from build123d import *

# Parameters (mm, degrees)
SKETCH1_R                = 5
BOSS_EXTRUDE1_DEPTH      = 1.5
BOSS_EXTRUDE1_DEPTH_BACK = 1.5


with BuildPart() as part:
    # Sketch1 → Boss-Extrude1 (new body, two sides)
    with BuildSketch(Plane.XY) as boss_extrude1_sk:
        with BuildLine():
            Line((-12.7, 0), (-12.7, -30.012513048))
            Line((-12.7, -30.012513048), (-11.2, -30.012513048))
            ThreePointArc((-11.2, -30.012513048), (0, -23.3), (11.2, -30.012513048))
            Line((11.2, -30.012513048), (12.7, -30.012513048))
            Line((12.7, -30.012513048), (12.7, 0))
            ThreePointArc((12.7, 0), (0, 12.7), (-12.7, 0))
        make_face()
        Circle(SKETCH1_R, mode=Mode.SUBTRACT)
    extrude(amount=BOSS_EXTRUDE1_DEPTH)
    extrude(boss_extrude1_sk.sketch, amount=-BOSS_EXTRUDE1_DEPTH_BACK)


solid = part.part
The listing builds one solid part. Answer for the finished solid, in the listing's coordinates (mm). Round coordinates to 2 decimals unless told otherwise and drop trailing zeros. Write each loop counter-clockwise with the first axis right and the second up, starting at its lowest first coordinate (ties: lowest second). Pieces come first, ordered by that corner, then holes. Notation, with made-up numbers: M -4.5,-6.5 L 37.5,-6.5 A23 ccw 37.5,29.5 Z; hole C -36.5,-31.5 d8. An arc over 180 degrees is marked long. Write each question's results on one line, items separated by ' | '. Start each with the question number.
(1) The part is cut by section A-A, the plane z = -0.05. Write down the section's boundary in (x, y).
(2) This flat-tipped pin is pushed along its axis until it touches: P1, Ø1, axis at y = 3.5, z = 0, coming from the +X side. Where does it stop, or does it pass through?
(3) The part is cut by section B-B, the plane x = 0. Write down the section's boundary in (y, z), and give its area (3 significant figures).
(4) The part is cut by section D-D, the plane y = 7.5. Write down the section's boundary in (x, z).
(5) Find the intervals of material crossed by line 1 (X direction, y = -27.5, z = -1.15); line 2 (Y direction, x = 4, z = -0.55); line 3 (X direction, y = 1, z = -0.45), in increasing order.
(6) Determine the mould class of faces 1 (the cylindrical face through (-1.08, -4.88, -0.02)), 2 (the flat face through (12, -30.013, 0)), 3 (the flat face through (12.7, -15, 0)) for opening direction Y: +Y half, -Y half, draft (parallel to the pull), parting line (faces both ways), or undercut.
(7) The part is cut by section C-C, the plane y = 1.5. Write down the section's boundary in (x, z), and give its area (3 significant figures).
Worked answers:
1) outline: M -12.7,-30.01 L -11.2,-30.01 A12.7 cw 11.2,-30.01 L 12.7,-30.01 L 12.7,0 A12.7 ccw -12.7,0 Z; hole C 0,0 d10
2) P1: stops at x = 12.34
3) outline: M -23.3,-1.5 L -5,-1.5 L -5,1.5 L -23.3,1.5 Z; M 5,-1.5 L 12.7,-1.5 L 12.7,1.5 L 5,1.5 Z | area: 78.0 mm²
4) outline: M -10.25,-1.5 L 10.25,-1.5 L 10.25,1.5 L -10.25,1.5 Z
5) line 1: x = -12.7 to -9.44, 9.44 to 12.7 | line 2: y = -23.95 to -3, 3 to 12.05 | line 3: x = -12.66 to -4.9, 4.9 to 12.66
6) face 1: undercut | face 2: -Y half | face 3: draft
7) outline: M -12.61,-1.5 L -4.77,-1.5 L -4.77,1.5 L -12.61,1.5 Z; M 4.77,-1.5 L 12.61,-1.5 L 12.61,1.5 L 4.77,1.5 Z | area: 47.0 mm²
